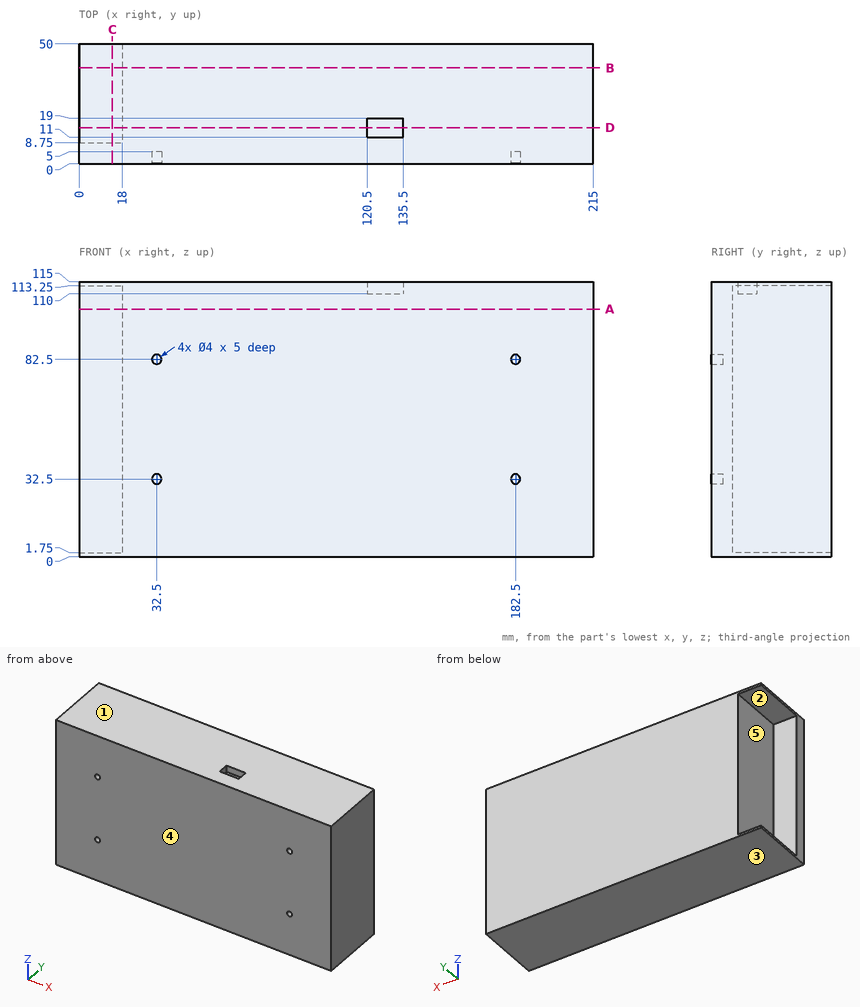
Geometry: see drawing. Coordinates: mm, zero at the bounding-box minimum. A direction names the side the tool comes from. Give positions to 0.01 mm unless a question says otherwise; leave off trailing zeros. Loops run counter-clockwise (first coordinate to the right, second up) from the corner with the lowest first, then second, coordinate; pieces in that order, holes last. Notation, with made-up numbers: (89.5, 71) - (141.5, 71) arc R26 cw to (141.5, 91) - close; hole circle Ø9 at (71, -5.75). An arc over 180 degrees is marked (long way). Answer as CSV lines item,"result". Start each with the question number.
1. Section D-D, the plane y = 15. Return loops of the section in (x, z).
2. Ray query, L1, parallel to X at y = 2.55, z = 32.5; L2, parallel to Z at x = 32, y = 3; L3, parallel to X at y = 21.5, z = 106.5. Return the intervals inside material, ascending.
3. Section A-A, the plane z = 103.5. Return loops of the section in (x, y), plus the area to 3 significant figures.
4. Section C-C, the plane x = 14. Return loops of the section in (y, z).
5. Reachability of the marked faces 4 and 5 from +Z, -Z, +X, -X, +Y, -Y: full face, straight path, thin tool, end or side. Return the list, or none.
6. Draft query along Z for the marked faces 1, 2 and 3. Return one class per face: released by +Z, released by -Z, zero draft, split by the parting line, or undercut.
7. Pin query (flat end, axial travel): P1, Ø2.5, axis at x = 182.5, z = 32.5, coming from the -Y side; P2, Ø3, axis at y = 38, z = 96.5, coming from the -X side; P3, Ø14.5, axis at x = 7.5, z = 46.5, coming from the +Y side. Return the tip coordinate at first contact, or that it passes through.
8. Section B-B, the plane y = 40. Return loops of the section in (x, z), plus the area to 3 significant figures.
Answers:
1,outline,"(0, 0) - (215, 0) - (215, 115) - (135.5, 115) - (135.5, 110) - (120.5, 110) - (120.5, 115) - (0, 115) - (0, 113.25) - (18, 113.25) - (18, 1.75) - (0, 1.75) - close"
2,L1,"x = 0 to 30.5, 34.5 to 180.5, 184.5 to 215"
2,L2,"z = 0 to 30.56, 34.44 to 80.56, 84.44 to 115"
2,L3,"x = 18 to 215"
3,outline,"(0, 0) - (215, 0) - (215, 50) - (18, 50) - (18, 8.75) - (0, 8.75) - close"
3,area,"10,000 mm2"
4,outline,"(0, 0) - (50, 0) - (50, 1.75) - (8.75, 1.75) - (8.75, 113.25) - (50, 113.25) - (50, 115) - (0, 115) - close"
5,face 4,"+Z, -Z, +X, -X, -Y"
5,face 5,"-X, +Y"
6,face 1,"released by +Z"
6,face 2,"undercut"
6,face 3,"released by -Z"
7,P1,"stops at y = 5"
7,P2,"stops at x = 18"
7,P3,"stops at y = 8.75"
8,outline,"(0, 0) - (215, 0) - (215, 115) - (0, 115) - (0, 113.25) - (18, 113.25) - (18, 1.75) - (0, 1.75) - close"
8,area,"22,700 mm2"
